Could you check a few things on this model? Use its own coordinates, in mm. Coordinates: 2 decimals unless noted, no trailing zeros. Write each loop counter-clockwise with the first axis right and the second up, starting at its lowest first coordinate (ties: lowest second). Pieces come first, ordered by that corner, then holes. Notation, with made-up numbers: (-35.75, 4) - (3.25, 4) arc R19 cw to (3.25, 37) - close; hole circle Ø3 at (60.25, 67). An arc over 180 degrees is marked (long way). Answer as a JSON object with one key per item and string values. Group by question number.
1) Will these pins go through, and if not, where does the flat tip stop? pin 1 Ø1 at (x, y) = (12.5, 0.5) entering from +Z; pin 2 Ø0.8 at (x, y) = (12.5, 1.5) entering from -Z; pin 3 Ø1.1 at (y, z) = (1.5, -25.5) entering from -X; pin 4 Ø22 at (x, z) = (17, -17) entering from +Y.
2) If we section it at C-C (z = -16): Write out the boundary of the cut face in (x, y), plus the area to 3 significant figures.
3) We'd pull the mould along Z, two halves only. Please class faces 1 (the flat face through (19, 1, -30)), 2 (the flat face through (17, 0, -30)), 3 (the cylindrical face through (17.26, 0.58, -0.85)): released by +Z, released by -Z, zero draft, split by the parting line, or undercut.
4) If we section it at B-B (x = 2.5): Write out the boundary of the cut face in (y, z), plus the area to 3 significant figures.
5) If we section it at D-D (y = 1.6): State how many separate pieces and enclosed holes the cut face has, plus the area to 3 significant figures.
6) Please list where these lines run through material, in increasing order: line 1 along X through (y, z) = (0.7, -57.5); line 2 along Z through (x, y) = (2.5, 0.65); line 3 along Z through (x, y) = (2.5, 1).
7) If we section it at A-A (x = 16): Write out the boundary of the cut face in (y, z), plus the area to 3 significant figures.
```python
from build123d import *

# Parameters (mm, degrees)
SKETCH1_W           = 37.5
SKETCH1_H           = 60
BOSS_EXTRUDE1_DEPTH = 2
SKETCH2_R           = 1
CUT_EXTRUDE1_DEPTH  = 71.783119457
SKETCH3_W           = 27.5
SKETCH3_H           = 56
CUT_EXTRUDE2_DEPTH  = 1
FILLET1_R           = 2.5
FILLET2_R           = 2.5


with BuildPart() as part:
    # Sketch1 → Boss-Extrude1 (new body)
    with BuildSketch(Plane(origin=(0, 0, 0), x_dir=(1, 0, 0), z_dir=(0, 1, 0))):
        with Locations((18.75, 30)):
            Rectangle(SKETCH1_W, SKETCH1_H)
    extrude(amount=BOSS_EXTRUDE1_DEPTH)

    # Sketch2 → Cut-Extrude1 (cut, through all)
    with BuildSketch(Plane(origin=(0, 2, 0), x_dir=(1, 0, 0), z_dir=(0, 1, 0))):
        with Locations(Location((2.5, 57.5, 0), (0, 0, 270))):
            Circle(SKETCH2_R)
        with Locations(Location((35, 57.5, 0), (0, 0, 270))):
            Circle(SKETCH2_R)
        with Locations(Location((35, 2.5, 0), (0, 0, 270))):
            Circle(SKETCH2_R)
        with Locations(Location((2.5, 2.5, 0), (0, 0, 270))):
            Circle(SKETCH2_R)
    extrude(amount=-CUT_EXTRUDE1_DEPTH, mode=Mode.SUBTRACT)

    # Sketch3 → Cut-Extrude2 (cut)
    with BuildSketch(Plane(origin=(0, 2, 0), x_dir=(1, 0, 0), z_dir=(0, 1, 0))):
        with Locations((18.75, 30)):
            Rectangle(SKETCH3_W, SKETCH3_H)
    extrude(amount=-CUT_EXTRUDE2_DEPTH, mode=Mode.SUBTRACT)

    # Fillet1
    fillet1_edges = [part.edges().sort_by_distance(p)[0] for p in [
        (37.5, 1, -60),
        (37.5, 1, 0),
    ]]
    fillet(fillet1_edges, radius=FILLET1_R)

    # Fillet2
    # the kernel refuses this fillet: 2.5 mm, written as the material it takes off along each edge
    with BuildSketch(Plane(origin=(35, 0, -60), x_dir=(0, 0, 1), z_dir=(-1, 0, 0))) as fillet2_piece_1:
        with BuildLine():
            CenterArc((2.449489743, 2.5), FILLET2_R, 191.536959033, 78.463040967)
            Line((0, 2), (0, 0))
            Line((0, 0), (2.449489743, 0))
        make_face()
    extrude(amount=41.123724357, mode=Mode.SUBTRACT)
    with BuildSketch(Plane(origin=(37.5, 0, -2.5), x_dir=(-1, 0, 0), z_dir=(0, 0, -1))) as fillet2_piece_2:
        with BuildLine():
            CenterArc((2.449489743, 2.5), FILLET2_R, 191.536959033, 78.463040967)
            Line((0, 2), (0, 0))
            Line((0, 0), (2.449489743, 0))
        make_face()
    extrude(amount=55, mode=Mode.SUBTRACT)
    with BuildSketch(Plane(origin=(-6.123724357, 0, 0), x_dir=(0, 1.0, -1.574296248917966e-12), z_dir=(1, 0, 0))) as fillet2_piece_3:
        with BuildLine():
            CenterArc((2.5, -2.449489743), FILLET2_R, 101.536959033, 78.463040967)
            Line((0, -2.449489743), (0, 0))
            Line((0, 0), (2, 0))
        make_face()
    extrude(amount=41.123724357, mode=Mode.SUBTRACT)
    with BuildSketch(Plane(origin=(35, 0, -2.5), x_dir=(0, 0, 1), z_dir=(-1, 0, 0))) as fillet2_piece_4:
        with BuildLine():
            CenterArc((0.050510257, 2.5), FILLET2_R, 270, 78.463040967)
            Line((2.5, 2), (2.5, 0))
            Line((2.5, 0), (0.050510257, 0))
        make_face()
    revolve(axis=Axis((35, 0, -2.5), (0, 1, 0)), revolution_arc=90, mode=Mode.SUBTRACT)
    with BuildSketch(Plane(origin=(35, 0, -57.5), x_dir=(1, 0, 0), z_dir=(0, 0, 1))) as fillet2_piece_5:
        with BuildLine():
            CenterArc((0.050510257, 2.5), FILLET2_R, 270, 78.463040967)
            Line((2.5, 2), (2.5, 0))
            Line((2.5, 0), (0.050510257, 0))
        make_face()
    revolve(axis=Axis((35, 0, -57.5), (0, 1, 0)), revolution_arc=90, mode=Mode.SUBTRACT)


solid = part.part
```
Here are the results:
{
 "1": {"pin 1": "stops at z = -0.45", "pin 2": "stops at z = -59.98", "pin 3": "stops at x = 0", "pin 4": "stops at y = 1"},
 "2": {"outline": "(0, 0) - (35.05, 0) arc R2.5 ccw to (37.5, 2) - (32.5, 2) - (32.5, 1) - (5, 1) - (5, 2) - (0, 2) - close", "area": "46.3 mm²"},
 "3": {"face 1": "undercut", "face 2": "zero draft", "face 3": "released by +Z"},
 "4": {"outline": "(0, -56.5) - (2, -56.5) - (2, -3.5) - (0, -3.5) - close; (0.19, -58.5) arc R2.5 ccw to (2, -60) - (2, -58.5) - close; (0.19, -1.5) - (2, -1.5) - (2, 0) arc R2.5 ccw to start", "area": "110 mm²"},
 "5": {"separate pieces": "1", "enclosed holes": "5", "area": "679 mm²"},
 "6": {"line 1": "x = 0 to 1.5, 3.5 to 34, 36 to 36.79", "line 2": "z = -59.23 to -58.5, -56.5 to -3.5, -1.5 to -0.77", "line 3": "z = -59.55 to -58.5, -56.5 to -3.5, -1.5 to -0.45"},
 "7": {"outline": "(0, -57.55) arc R2.5 ccw to (2, -60) - (2, -58) - (1, -58) - (1, -2) - (2, -2) - (2, 0) arc R2.5 ccw to (0, -2.45) - close", "area": "61.5 mm²"}
}
